Input: part model. Units: mm. Frame: model coordinates. Give positions to 0.01 mm unless a question says otherwise; leave off trailing zeros. Loops run counter-clockwise (first coordinate to the right, second up) from the corner with the lowest first, then second, coordinate; pieces in that order, holes last. Notation, with made-up numbers: M 18.5,3 L 47.5,3 A12 ccw 47.5,18 Z; hole C -21,49.5 d3. An arc over 180 degrees is marked long. Return JSON: item names as keys, results as strings. Group by question number.
```python
from build123d import *

# Parameters (mm, degrees)
SKETCH_W     = 40.07407
SKETCH_H     = 40.074074
PAD_DEPTH    = 15
SKETCH001_R  = 8.083249
POCKET_DEPTH = 15.001
FILLET_R     = 8


with BuildPart() as part:
    # Sketch → Pad (new body)
    with BuildSketch(Plane.XY):
        with Locations((20.037035, 20.037037)):
            Rectangle(SKETCH_W, SKETCH_H)
    extrude(amount=PAD_DEPTH)

    # Sketch001 (on Face6 of Pad) → Pocket (cut, through all)
    with BuildSketch(Plane.XY.offset(15)):
        with Locations((20.074074, 19.925928)):
            Circle(SKETCH001_R)
    extrude(amount=-POCKET_DEPTH, mode=Mode.SUBTRACT)

    # Fillet
    fillet_edges = [part.edges().sort_by_distance(p)[0] for p in [
        (40.07407, 0, 7.5),
        (40.07407, 40.074074, 7.5),
        (0, 40.074074, 7.5),
        (0, 0, 7.5),
    ]]
    fillet(fillet_edges, radius=FILLET_R)


solid = part.part
```
Item 1: Pull-direction query (X, two-part tool) for faces 1 (the face through (37.67, 37.79, 7.6)), 2 (the face through (20, 40.074, 7)), 3 (the face through (2.281, 37.668, 7.605)), 4 (the face through (14.12, 25.39, 7.6)); classes: pulls with the +X half, pulls with the -X half, needs draft (parallel to the pull), parting line crosses it, or undercut.
Item 2: Section D-D, the plane x = 3.5. Return loops of the section in (y, z).
Item 3: Section B-B, the plane x = 25. Return loops of the section in (y, z), then the cut area to 3 significant figures.
Item 4: Section A-A, the plane y = 26.5. Return loops of the section in (x, z), then the cut area to 3 significant figures.
Item 5: Material intervals for line 1 (Y direction, x = 22.5, z = 13); line 2 (Y direction, x = 15.5, z = 11); line 3 (X direction, y = 26, z = 11), sorted ascending. Write a range as from..to.
Item 6: Section C-C, the plane z = 9. Return loops of the section in (x, y).
Answer below:
{
 "1": {"face 1": "pulls with the +X half", "face 2": "needs draft", "face 3": "pulls with the -X half", "face 4": "undercut"},
 "2": {"outline": "M 1.39,0 L 38.69,0 L 38.69,15 L 1.39,15 Z"},
 "3": {"outline": "M 0,0 L 13.52,0 L 13.52,15 L 0,15 Z; M 26.33,0 L 40.07,0 L 40.07,15 L 26.33,15 Z", "area": "409 mm^2"},
 "4": {"outline": "M 0,0 L 15.37,0 L 15.37,15 L 0,15 Z; M 24.78,0 L 40.07,0 L 40.07,15 L 24.78,15 Z", "area": "460 mm^2"},
 "5": {"line 1": "0..12.22, 27.64..40.07", "line 2": "0..13.26, 26.59..40.07", "line 3": "0..14.74, 25.41..40.07"},
 "6": {"outline": "M 0,8 A8 ccw 8,0 L 32.07,0 A8 ccw 40.07,8 L 40.07,32.07 A8 ccw 32.07,40.07 L 8,40.07 A8 ccw 0,32.07 Z; hole C 20.07,19.93 d16.17"}
}
